Input: part model. Units: mm. Frame: model coordinates. A direction names the side the tool comes from. Give positions to 0.01 mm unless a question says otherwise; leave off trailing zeros. Loops run counter-clockwise (first coordinate to the right, second up) from the corner with the lowest first, then second, coordinate; pieces in that order, holes last. Notation, with made-up numbers: M 15.25,53 L 40.25,53 A28 cw 40.25,85 Z; hole C -37.5,25.5 d5. An arc over 180 degrees is marked long. Use CSV: the item, a comma, the result in double quotes. Start each with the question number.
Q1. Section B-B, the plane y = -12.5. Output: boundary loops of the cut face in (x, z), plus the area to 3 significant figures.
Q2. Pull-direction query (X, two-part tool) for faces 6 (the cylindrical face through (22.734, -15.72, 14.824)), 7 (the flat face through (12, 25, 0)), 8 (the flat face through (40, -3, 4)), 9 (the cylindrical face through (-42, 36, 5)); classes: released by +X, released by -X, zero draft, split by the parting line, or undercut.
Q3. Pin query (flat end, axial travel): pin 1 (12 mm diameter, centred on x = 17, z = 34, fed in from -Y); pin 2 (12 mm diameter, centred on y = -5.5, z = 6, fed in from -X); pin 3 (5 mm diameter, centred on x = 12.5, z = 28, fed in from -Y); pin 4 (3.5 mm diameter, centred on x = -43.5, z = 7, fed in from +Y). Return the tip coordinate at first contact, or that it passes through.
Q4. Section C-C, the plane x = -52. Output: boundary loops of the cut face in (y, z).
Q5. Material intervals for line 1 along Y through (x, z) = (-49, 23); line 2 along Y through (x, z) = (-32, 22.5); line 3 along Z through (x, y) = (13.5, -16), sorted ascending.
Q6. Section D-D, the plane y = 44. Output: boundary loops of the cut face in (x, z).
Q7. Section A-A, the plane z = 15. Output: boundary loops of the cut face in (x, y).
Q8. Reachability of faces 1 (the flat face through (-38, 56.675, 4)), 2 (the flat face through (15, 9, 14)), 3 (the flat face through (0, 5, 15)), 4 (the flat face through (20, -23.325, 12)), 5 (the flat face through (11, -6, 25)) from +Z, -Z, +X, -X, +Y, -Y: full face, straight path, thin tool, end or side. Return the list, or none.
from build123d import *

# Parameters (mm, degrees)
BOSS_EXTRUDE1_DEPTH     = 40
SKETCH2_R               = 4
CUT_EXTRUDE1_DEPTH      = 30
SKETCH3_R               = 6.5
CUT_EXTRUDE2_DEPTH      = 100
CUT_EXTRUDE2_DEPTH_BACK = 100
SKETCH5_W               = 35
SKETCH5_H               = 20
CUT_EXTRUDE3_DEPTH      = 60
SKETCH6_W               = 5
SKETCH6_H               = 65
BOSS_EXTRUDE2_DEPTH     = 25
CUT_EXTRUDE4_DEPTH      = 10
FILLET1_R               = 10
SKETCH8_W               = 40
SKETCH8_H               = 48
CUT_EXTRUDE5_DEPTH      = 15
FILLET2_R               = 5


with BuildPart() as part:
    # Sketch1 → Boss-Extrude1 (new body)
    with BuildSketch(Plane.XY):
        Polygon((40, -23.325428286), (0, -23.325428286), (0, 34.674571714), (-59, 34.674571714), (-59, 56.674571714), (15, 56.674571714), (15, -8.325428286), (40, -8.325428286), align=None)
    extrude(amount=BOSS_EXTRUDE1_DEPTH)

    # Sketch2 → Cut-Extrude1 (cut)
    with BuildSketch(Plane(origin=(0, -8.325428286, 0), x_dir=(1, 0, 0), z_dir=(0, 1, 0))):
        with Locations((26.730150284, -15)):
            Circle(SKETCH2_R)
    extrude(amount=-CUT_EXTRUDE1_DEPTH, mode=Mode.SUBTRACT)

    # Sketch3 → Cut-Extrude2 (cut, two sides)
    with BuildSketch(Plane(origin=(-59, 0, 0), x_dir=(0, 0, -1), z_dir=(1, 0, 0))) as cut_extrude2_sk:
        with Locations((-23, 46.674571714)):
            Circle(SKETCH3_R)
    extrude(amount=CUT_EXTRUDE2_DEPTH, mode=Mode.SUBTRACT)
    extrude(cut_extrude2_sk.sketch, amount=-CUT_EXTRUDE2_DEPTH_BACK, mode=Mode.SUBTRACT)

    # Sketch5 → Cut-Extrude3 (cut)
    with BuildSketch(Plane(origin=(15, 0, 0), x_dir=(0, 0, -1), z_dir=(1, 0, 0))):
        with Locations((-22.5, 46.674571714)):
            Rectangle(SKETCH5_W, SKETCH5_H)
    extrude(amount=-CUT_EXTRUDE3_DEPTH, mode=Mode.SUBTRACT)

    # Sketch6 → Boss-Extrude2 (add)
    with BuildSketch(Plane(origin=(15, 0, 0), x_dir=(0, 0, -1), z_dir=(1, 0, 0))):
        with Locations((-2.5, 24.174571714)):
            Rectangle(SKETCH6_W, SKETCH6_H)
    extrude(amount=BOSS_EXTRUDE2_DEPTH)

    # Sketch7 → Cut-Extrude4 (cut)
    with BuildSketch(Plane(origin=(0, 36.674571714, 0), x_dir=(1, 0, 0), z_dir=(0, 1, 0))):
        with BuildLine():
            Line((-39, -8), (-39, -34))
            ThreePointArc((-39, -34), (-42, -37), (-45, -34))
            Line((-45, -34), (-45, -8))
            ThreePointArc((-45, -8), (-42, -5), (-39, -8))
        make_face()
    extrude(amount=-CUT_EXTRUDE4_DEPTH, mode=Mode.SUBTRACT)

    # Fillet1
    fillet1_edges = [part.edges().sort_by_distance(p)[0] for p in [
        (15, 36.674571714, 22.5),
        (40, 56.674571714, 2.5),
    ]]
    fillet(fillet1_edges, radius=FILLET1_R)

    # Sketch8 → Cut-Extrude5 (cut)
    with BuildSketch(Plane.XY.offset(40)):
        with Locations((20, 0.674571714)):
            Rectangle(SKETCH8_W, SKETCH8_H)
    extrude(amount=-CUT_EXTRUDE5_DEPTH, mode=Mode.SUBTRACT)

    # Fillet2
    fillet2_edges = [part.edges().sort_by_distance(p)[0] for p in [
        (7.5, 24.674571714, 40),
        (7.5, 24.674571714, 25),
    ]]
    fillet(fillet2_edges, radius=FILLET2_R)


solid = part.part
A:
1,outline,"M 0,0 L 40,0 L 40,25 L 0,25 Z; hole C 26.73,15 d8"
1,area,"950 mm^2"
2,face 6,"undercut"
2,face 7,"zero draft"
2,face 8,"released by +X"
2,face 9,"undercut"
3,pin 1,"y = 24.39"
3,pin 2,"x = 0"
3,pin 3,"y = 21.85"
3,pin 4,"y = 56.67"
4,outline,"M 34.67,0 L 56.67,0 L 56.67,40 L 34.67,40 Z; hole C 46.67,23 d13"
5,line 1,"34.67 to 40.17, 53.17 to 56.67"
5,line 2,"34.67 to 36.67"
5,line 3,"0 to 25"
6,outline,"M -59,0 L 40,0 L 40,5 L -45,5 L -45,17.08 L -59,17.08 Z; M -59,28.92 L -45,28.92 L -45,40 L -59,40 Z"
7,outline,"M -59,34.67 L -45,34.67 L -45,56.67 L -59,56.67 Z; M -39,34.67 L 0,34.67 L 0,-23.33 L 22.73,-23.33 L 22.73,-8.33 L 15,-8.33 L 15,26.67 A10 ccw 5,36.67 L -39,36.67 Z; M 30.73,-23.33 L 40,-23.33 L 40,-8.33 L 30.73,-8.33 Z"
8,face 1,"+Z, -Z, +X, -X, +Y"
8,face 2,"+Z, +X, +Y"
8,face 3,"+Z, -Z, -X, -Y"
8,face 4,"+Z, -Z, +X, -X, -Y"
8,face 5,"+Z, +X, -X, -Y"
